from build123d import *

# Parameters (mm, degrees)
SKETCH1_W               = 85
SKETCH1_H               = 56
BOSS_EXTRUDE1_DEPTH     = 3.175
SKETCH2_R               = 6.35
CUT_EXTRUDE1_DEPTH      = 3.175
SKETCH3_R               = 1.778
CUT_EXTRUDE2_DEPTH      = 3.175
CIRPATTERN1_COUNT       = 4
SKETCH4_R               = 3
BOSS_EXTRUDE2_DEPTH     = 6.35
SKETCH6_R               = 1.349999967
CUT_EXTRUDE3_DEPTH      = 7.35
CUT_EXTRUDE3_DEPTH_BACK = 4.175
SKETCH7_R               = 2.159
CUT_EXTRUDE4_DEPTH      = 7.025
SKETCH8_W               = 19.05
SKETCH8_H               = 38.1
CUT_EXTRUDE5_DEPTH      = 1.5875
FILLET1_R               = 2.032


with BuildPart() as part:
    # Sketch1 → Boss-Extrude1 (new body)
    with BuildSketch(Plane.XY):
        with Locations((42.5, 28)):
            Rectangle(SKETCH1_W, SKETCH1_H)
    extrude(amount=BOSS_EXTRUDE1_DEPTH)

    # Sketch2 → Cut-Extrude1 (cut)
    with BuildSketch(Plane.XY.offset(3.175)):
        with Locations((42.5, 28)):
            Circle(SKETCH2_R)
    extrude(amount=-CUT_EXTRUDE1_DEPTH, mode=Mode.SUBTRACT)

    # Sketch3 → Cut-Extrude2 (cut)
    with BuildSketch(Plane.XY.offset(3.175)):
        with Locations((42.5, 37.779)):
            Circle(SKETCH3_R)
    cut_extrude2 = extrude(amount=-CUT_EXTRUDE2_DEPTH, mode=Mode.SUBTRACT)

    # CirPattern1: Cut-Extrude2 ×4 about axis
    cirpattern1_axis = Axis((42.5, 28, 0), (0, 0, 1))
    for i in range(1, CIRPATTERN1_COUNT):
        add(cut_extrude2.rotate(cirpattern1_axis, i * 360 / CIRPATTERN1_COUNT), mode=Mode.SUBTRACT)

    # Sketch4 → Boss-Extrude2 (add)
    with BuildSketch(Plane.XY.offset(3.175)):
        with Locations((3.5, 52.5)):
            Circle(SKETCH4_R)
        with Locations((3.5, 3.5)):
            Circle(SKETCH4_R)
        with Locations((61.5, 52.5)):
            Circle(SKETCH4_R)
        with Locations((61.5, 3.5)):
            Circle(SKETCH4_R)
    extrude(amount=BOSS_EXTRUDE2_DEPTH)

    # Sketch6 → Cut-Extrude3 (cut, two sides)
    with BuildSketch(Plane.XY.offset(3.175)) as cut_extrude3_sk:
        with Locations((3.5, 3.5)):
            Circle(SKETCH6_R)
        with Locations((61.5, 3.5)):
            Circle(SKETCH6_R)
        with Locations((61.5, 52.5)):
            Circle(SKETCH6_R)
        with Locations((3.5, 52.5)):
            Circle(SKETCH6_R)
    extrude(amount=CUT_EXTRUDE3_DEPTH, mode=Mode.SUBTRACT)
    extrude(cut_extrude3_sk.sketch, amount=-CUT_EXTRUDE3_DEPTH_BACK, mode=Mode.SUBTRACT)

    # Sketch7 → Cut-Extrude4 (cut)
    with BuildSketch(Plane(origin=(0, 0, 0), x_dir=(-1, 0, 0), z_dir=(0, 0, -1))):
        with Locations((-61.5, 52.5)):
            Circle(SKETCH7_R)
        with Locations((-3.5, 52.5)):
            Circle(SKETCH7_R)
        with Locations((-3.5, 3.5)):
            Circle(SKETCH7_R)
        with Locations((-61.5, 3.5)):
            Circle(SKETCH7_R)
    extrude(amount=-CUT_EXTRUDE4_DEPTH, mode=Mode.SUBTRACT)

    # Sketch8 → Cut-Extrude5 (cut)
    with BuildSketch(Plane.XY.offset(3.175)):
        with Locations((19.05, 28)):
            Rectangle(SKETCH8_W, SKETCH8_H)
        with Locations((65.95, 28)):
            Rectangle(SKETCH8_W, SKETCH8_H)
    extrude(amount=-CUT_EXTRUDE5_DEPTH, mode=Mode.SUBTRACT)

    # Fillet1
    fillet1_edges = [part.edges().sort_by_distance(p)[0] for p in [
        (9.525, 8.95, 2.38125),
        (9.525, 47.05, 2.38125),
        (28.575, 47.05, 2.38125),
        (28.575, 8.95, 2.38125),
        (56.425, 8.95, 2.38125),
        (56.425, 47.05, 2.38125),
        (75.475, 47.05, 2.38125),
        (75.475, 8.95, 2.38125),
        (0, 56, 1.5875),
        (85, 56, 1.5875),
        (85, 0, 1.5875),
        (0, 0, 1.5875),
    ]]
    fillet(fillet1_edges, radius=FILLET1_R)


solid = part.part
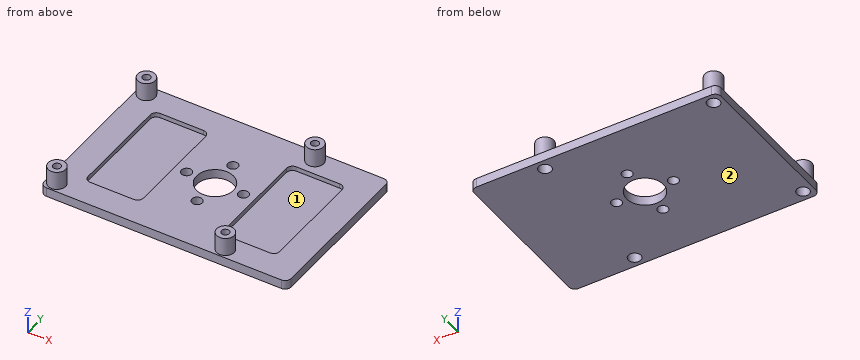
Verification items for the finished model (mm, model axes). Face numbers are marked on the shaded views. Coordinates: 2 decimals unless noted, no trailing zeros. Order: outer loops, then holes, each group sorted by start corner. A loop starts at its lowest first (then second) coordinate and runs counter-clockwise, first axis right, second up.
1. Release check for a two-part mould opening along Y. For the marked faces 1 and 2 record: +Y half, -Y half, draft (parallel to the pull), parting line (faces both ways), or undercut.
Results found:
face 1: undercut
face 2: draft
2. Sectioned sample at A-A, the plane z = 5.25. Record the cut outline in (x, y), and give its area (3 significant figures).
Results found:
outline: circle Ø6 at (3.5, 3.5); circle Ø6 at (3.5, 52.5); circle Ø6 at (61.5, 3.5); circle Ø6 at (61.5, 52.5); hole circle Ø4.32 at (3.5, 3.5); hole circle Ø4.32 at (3.5, 52.5); hole circle Ø4.32 at (61.5, 3.5); hole circle Ø4.32 at (61.5, 52.5)
area: 54.5 mm2
3. Sectioned sample at C-C, the plane x = 3.5. Record the cut outline in (y, z) (3 decimals), and give its area (3 significant figures).
Results found:
outline: (0, 0) - (1.341, 0) - (1.341, 7.025) - (2.15, 7.025) - (2.15, 9.525) - (0.5, 9.525) - (0.5, 3.175) - (0, 3.175) - close; (4.85, 7.025) - (5.659, 7.025) - (5.659, 0) - (50.341, 0) - (50.341, 7.025) - (51.15, 7.025) - (51.15, 9.525) - (49.5, 9.525) - (49.5, 3.175) - (6.5, 3.175) - (6.5, 9.525) - (4.85, 9.525) - close; (53.85, 7.025) - (54.659, 7.025) - (54.659, 0) - (56, 0) - (56, 3.175) - (55.5, 3.175) - (55.5, 9.525) - (53.85, 9.525) - close
area: 180 mm2
4. Go/stop test with flat-tipped pins: pin 1 Ø4.5 at (x, y) = (32.721, 28) entering from +Z (3 decimals); pin 2 Ø1.7 at (y, z) = (23, 3) entering from -X; pin 3 Ø5.5 at (x, y) = (22, 29.5) entering from +Z. Record where each tip stops, or that it passes through.
Results found:
pin 1: stops at z = 3.175
pin 2: stops at x = 0
pin 3: stops at z = 1.59
5. Sectioned sample at B-B, the plane y = 28. Give the number of separate pieces and of enclosed holes in the cut face, and give its area (3 significant figures).
Results found:
separate pieces: 4
enclosed holes: 0
area: 146 mm2
6. Sectioned sample at D-D, the plane y = 52.5. Record the cut outline in (x, z) (3 decimals), and give its area (3 significant figures).
Results found:
outline: (0, 0) - (1.341, 0) - (1.341, 7.025) - (2.15, 7.025) - (2.15, 9.525) - (0.5, 9.525) - (0.5, 3.175) - (0, 3.175) - close; (4.85, 7.025) - (5.659, 7.025) - (5.659, 0) - (59.341, 0) - (59.341, 7.025) - (60.15, 7.025) - (60.15, 9.525) - (58.5, 9.525) - (58.5, 3.175) - (6.5, 3.175) - (6.5, 9.525) - (4.85, 9.525) - close; (62.85, 7.025) - (63.659, 7.025) - (63.659, 0) - (85, 0) - (85, 3.175) - (64.5, 3.175) - (64.5, 9.525) - (62.85, 9.525) - close
area: 272 mm2
7. Scan lines: line 1 (X direction, y = 11.5, z = 2.5) (3 decimals); line 2 (Y direction, x = 3.5, z = 8.6); line 3 (Y direction, x = 3.5, z = 2.25). Record each from-to range of solid material in increasing order.
Results found:
line 1: x = 0 to 9.525, 28.575 to 56.425, 75.475 to 85
line 2: y = 0.5 to 2.15, 4.85 to 6.5, 49.5 to 51.15, 53.85 to 55.5
line 3: y = 0 to 1.34, 5.66 to 50.34, 54.66 to 56
